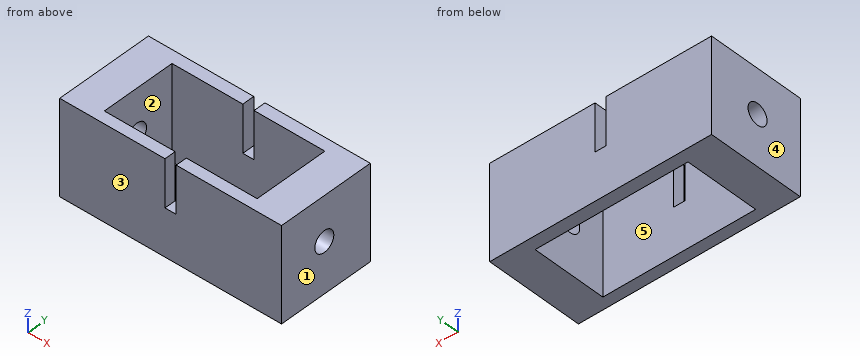
from build123d import *

# Parameters (mm, degrees)
F0_W     = 18.556535
F0_H     = 6.506839
F0_W_2   = 38.07705
F0_H_2   = 40.245993
F0_H_3   = 6.024849
F1_DEPTH = 50.8
F2_R     = 5.6515
F3_DEPTH = 170.688
F4_W     = 6.024849
F4_H     = 25.4
F5_DEPTH = 25.4
F6_W     = 6.506839
F6_H     = 25.4
F7_DEPTH = 25.4


with BuildPart() as f1:
    # F0 (on Top) → F1 (new body)
    with BuildSketch(Plane.XY):
        with Locations((-50.367742, 24.099397)):
            Rectangle(F0_W, F0_H)
        with Locations((-22.05095, 24.099397)):
            Rectangle(F0_W_2, F0_H)
        with Locations((-50.367742, 0.722981)):
            Rectangle(F0_W, F0_H_2)
        with Locations((-50.367742, -22.412439)):
            Rectangle(F0_W, F0_H_3)
        with Locations((-22.05095, -22.412439)):
            Rectangle(F0_W_2, F0_H_3)
    extrude(amount=F1_DEPTH)

    # F2 (on face) → F3 (cut)
    with BuildSketch(Plane(origin=(-59.64601, 0, 0), x_dir=(0, -1, 0), z_dir=(-1, 0, 0))):
        with Locations((0, 27.094796)):
            Circle(F2_R)
    extrude(amount=-F3_DEPTH, mode=Mode.SUBTRACT)

    # F4 (on face) → F5 (join)
    with BuildSketch(Plane.YZ.offset(-3.012425)):
        with Locations((-22.412439, 12.7)):
            Rectangle(F4_W, F4_H)
    extrude(amount=F5_DEPTH)

    # F6 (on face) → F7 (join)
    with BuildSketch(Plane.YZ.offset(-3.012425)):
        with Locations((24.099397, 12.7)):
            Rectangle(F6_W, F6_H)
    extrude(amount=F7_DEPTH)

    # F8: F1 across plane


with BuildPart() as f1_1:
    add(f1.part)
    add(f1.part.mirror(Plane.YZ))


solid = f1_1.part
Here's how the part is built. I have some questions about the finished solid (model axes, mm). Face numbers are marked on the shaded views. A direction names the side the tool comes from. Give positions to 0.01 mm unless a question says otherwise; leave off trailing zeros. Loops run counter-clockwise (first coordinate to the right, second up) from the corner with the lowest first, then second, coordinate; pieces in that order, holes last. Notation, with made-up numbers: (4.25, 76) -> (51.25, 76) arc R10 cw to (51.25, 94) -> close; hole circle Ø7 at (4, 32). An arc over 180 degrees is marked (long way). Answer as a JSON object with one key per item and string values. Group by question number.
Item 1: Thinking about a two-plate mould opening in X: for the marked faces 1, 2 and 3, which applies, pulls with the +X half, pulls with the -X half, needs draft (parallel to the pull), parting line crosses it, or undercut?
Item 2: Imagine slicing it at D-D on y = 10. Write out the boundary of the cut face in (x, z).
Item 3: Imagine slicing it at A-A on z = 42. Write out the boundary of the cut face in (x, y), then the cut area to 3 significant figures.
Item 4: Will these pins go through, and if not, where does the flat tip stop? pin 1 (5 mm diameter, centred on x = -37.5, y = 15, fed in from +Z); pin 2 (5 mm diameter, centred on x = -1.5, y = 24, fed in from +Z).
Item 5: On a 3-axis mill with a long thin cutter (end or side, diameter ignored), from which of +Z, -Z, +X, -X, +Y, -Y can I reach the whole of each face in a straight line? I mean the marked faces 4 and 5. Say none if no direction works.
Item 6: I need wall thicknesses on L1, parallel to X at y = 14.5, z = 10; L2, parallel to Z at x = 45.75, y = 0; L3, parallel to Y at x = -8, z = 18. Which ranges of each line are inside material? Lowest first, please.
Item 7: Imagine slicing it at C-C on x = 35.5. Write out the boundary of the cut face in (y, z).
Item 8: Imagine slicing it at B-B on y = 0. Write out the boundary of the cut face in (x, z).
Answer list:
{
 "1": {"face 1": "pulls with the +X half", "face 2": "undercut", "face 3": "needs draft"},
 "2": {"outline": "(-59.65, 0) -> (-41.09, 0) -> (-41.09, 50.8) -> (-59.65, 50.8) -> close; (41.09, 0) -> (59.65, 0) -> (59.65, 50.8) -> (41.09, 50.8) -> close"},
 "3": {"outline": "(-59.65, -25.42) -> (-3.01, -25.42) -> (-3.01, -19.4) -> (-41.09, -19.4) -> (-41.09, 20.85) -> (-3.01, 20.85) -> (-3.01, 27.35) -> (-59.65, 27.35) -> close; (3.01, -25.42) -> (59.65, -25.42) -> (59.65, 27.35) -> (3.01, 27.35) -> (3.01, 20.85) -> (41.09, 20.85) -> (41.09, -19.4) -> (3.01, -19.4) -> close", "area": "2,910 mm2"},
 "4": {"pin 1": "passes through", "pin 2": "stops at z = 50.8"},
 "5": {"face 4": "+Z, -Z, -X, +Y, -Y", "face 5": "+Z, -Z"},
 "6": {"L1": "x = -59.65 to -41.09, 41.09 to 59.65", "L2": "z = 0 to 21.44, 32.75 to 50.8", "L3": "y = -25.42 to -19.4, 20.85 to 27.35"},
 "7": {"outline": "(-25.42, 0) -> (-19.4, 0) -> (-19.4, 50.8) -> (-25.42, 50.8) -> close; (20.85, 0) -> (27.35, 0) -> (27.35, 50.8) -> (20.85, 50.8) -> close"},
 "8": {"outline": "(-59.65, 0) -> (-41.09, 0) -> (-41.09, 21.44) -> (-59.65, 21.44) -> close; (-59.65, 32.75) -> (-41.09, 32.75) -> (-41.09, 50.8) -> (-59.65, 50.8) -> close; (41.09, 0) -> (59.65, 0) -> (59.65, 21.44) -> (41.09, 21.44) -> close; (41.09, 32.75) -> (59.65, 32.75) -> (59.65, 50.8) -> (41.09, 50.8) -> close"}
}
